Design review of the part shown in the three views and the two pictorial views. Dimensions are in mm from the part's minimum x, y and z. A direction names the side the tool comes from. Give positions to 0.01 mm unless a question says otherwise; leave off trailing zeros. Write each loop counter-clockwise with the first axis right and the second up, starting at its lowest first coordinate (ties: lowest second). Pieces come first, ordered by that corner, then holes.
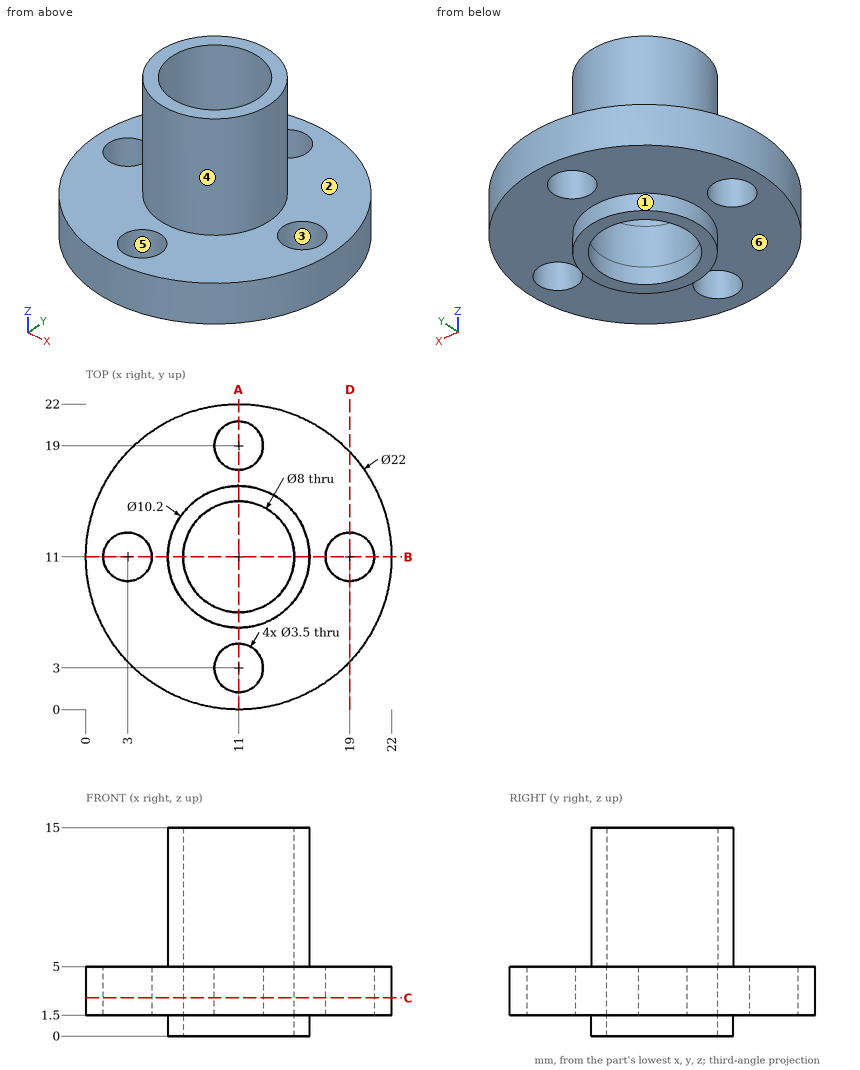
(1) Tool access review of the marked faces 1, 2 and 3: name each direction out of +Z, -Z, +X, -X, +Y, -Y from which nothing blocks a thin tool from reaching the whole face with its end or side.
Resolved:
face 1: -Z
face 2: +Z
face 3: +Z, -Z
(2) Consider section D-D, the plane x = 19. Give the boundary of the cut face in (y, z).
Resolved:
outline: (3.45, 1.5) - (9.25, 1.5) - (9.25, 5) - (3.45, 5) - close; (12.75, 1.5) - (18.55, 1.5) - (18.55, 5) - (12.75, 5) - close
(3) Mouldability with a two-part tool opening along X and no side actions: class the marked faces 4, 5 and 6 as pulls with the +X half, pulls with the -X half, needs draft (parallel to the pull), parting line crosses it, or undercut.
Resolved:
face 4: parting line crosses it
face 5: undercut
face 6: needs draft
(4) Clearance check with flat-ended pins moving along their axes: P1, Ø1, axis at y = 19.5, z = 2, coming from the -X side; P2, Ø8, axis at y = 3, z = 13.5, coming from the +X side; P3, Ø6, axis at y = 14, z = 12, coming from the +X side. State where each tip first meets the part, or that it passes through.
Resolved:
P1: stops at x = 3.45
P2: stops at x = 14.16
P3: stops at x = 16.1
(5) Consider section A-A, the plane x = 11. Give the boundary of the cut face in (y, z).
Resolved:
outline: (0, 1.5) - (1.25, 1.5) - (1.25, 5) - (0, 5) - close; (4.75, 1.5) - (5.9, 1.5) - (5.9, 0) - (7, 0) - (7, 15) - (5.9, 15) - (5.9, 5) - (4.75, 5) - close; (15, 0) - (16.1, 0) - (16.1, 1.5) - (17.25, 1.5) - (17.25, 5) - (16.1, 5) - (16.1, 15) - (15, 15) - close; (20.75, 1.5) - (22, 1.5) - (22, 5) - (20.75, 5) - close
(6) To check wall thickness, follow L1, parallel to Y at x = 11, z = 2.75; L2, parallel to Y at x = 11, z = 1.05; L3, parallel to Y at x = 12, z = 2. State the ranges of each line that lie inside material, in increasing order.
Resolved:
L1: y = 0 to 1.25, 4.75 to 7, 15 to 17.25, 20.75 to 22
L2: y = 5.9 to 7, 15 to 16.1
L3: y = 0.05 to 1.56, 4.44 to 7.13, 14.87 to 17.56, 20.44 to 21.95
(7) Consider section C-C, the plane z = 2.75. Give the boundary of the cut face in (x, y), then the cut area to 3 significant figures.
Resolved:
outline: circle Ø22 at (11, 11); hole circle Ø3.5 at (3, 11); hole circle Ø8 at (11, 11); hole circle Ø3.5 at (11, 3); hole circle Ø3.5 at (11, 19); hole circle Ø3.5 at (19, 11)
area: 291 mm2
